Check sheet for the modelled part. Datum: model origin and axes. Units: mm. Coordinates: 2 decimals unless noted, no trailing zeros. Order: outer loops, then holes, each group sorted by start corner. A loop starts at its lowest first (then second) coordinate and runs counter-clockwise, first axis right, second up. Notation, with made-up numbers: (18.25, 62.25) -> (32.25, 62.25) arc R26 ccw to (32.25, 78.25) -> close; hole circle Ø4 at (12, 60.25). An arc over 180 degrees is marked (long way). Put each result on its own line as item: value. Start each with the question number.
Autodesk Inventor part; units mm, degrees
ref_plane "YZ Plane" through (0, 0, 0) normal (1, 0, 0) x (0, 1, 0)
ref_plane "XZ Plane" through (0, 0, 0) normal (0, 1, 0) x (-1, 0, 0)
ref_plane "XY Plane" through (0, 0, 0) normal (0, 0, 1) x (1, 0, 0)
sketch "Náčrt1" plane through (0, 0, 0) normal (0, 0, 1) x (1, 0, 0)
  line L0 (-50, 25) -> (30, 25)
  line L1 (36.6643, -25) -> (-87.5, -25)
  line L2 (30, 25) -> (100, 0)
  line L3 (100, 0) -> (100, -25)
  line L4 (100, -25) -> (36.6643, -25)
  line L5 (-125, 0) -> (137.5, 0)
  line L6 (0, 35) -> (0, -35)
  line L7 (-50, 25) -> (-80, 0)
  line L8 (-80, 0) -> (-80, -25)
  line L9 (-80, -25) -> (-87.5, -25)
  point P0 (0, 0)
  point P1 (-35, 10)
  point P2 (15, 10)
  dimension "d0" = 50
  dimension "d2" = 80
  dimension "d3" = 25
  dimension "d4" = 50
  dimension "d6" = 15
  dimension "d16" = 70
  dimension "d17" = 30
  dimension "d18" = 25
  dimension "d19" = 50
  dimension "d20" = 35
  dimension "d21" = 25
  dimension "d22" = 25
extrude "Vysunutí1" add sketch "Náčrt1" along normal mid plane 4
hole "Díra1" at (-35, 10, 0) at (15, 10, 0) direction (0, 0, -1) diameter 6 end through all both
sketch "Náčrt2" plane through (0, 0, 2) normal (0, 0, 1) x (1, 0, 0)
  line L0 (-80, 0) -> (-80, -25)
  line L1 (-80, -25) -> (100, -25)
  line L2 (100, -25) -> (100, 0)
  point P0 (0, 0)
  point P1 (-40, -15)
  point P2 (60, -15)
  dimension "d23" = 40
  dimension "d24" = 10
  dimension "d25" = 40
  dimension "d26" = 10
hole "Díra2" at (-40, -15, 2) at (60, -15, 2) direction (0, 0, -1) diameter 3 depth 8
properties part number "Trup" material "Dřevo (Bříza)"
1) Sectioned sample at B-B (y = -15). Record the boundary of the cut face in (x, z), plus the area to 3 significant figures.
2) Mould release check, pull along X, two halves, no side actions. Record for faces 1 (the flat face through (-64.79, 12.675, -0.028)), 2 (the flat face through (9, 0, 2)), 3 (the cylindrical face through (17.93, 10.65, -0.03)): +X half, -X half, draft (parallel to the pull), parting line (faces both ways), or undercut.
3) Sectioned sample at C-C (z = -0.2). Record the boundary of the cut face in (x, y).
4) Sectioned sample at A-A (x = 15). Record the boundary of the cut face in (y, z), plus the area to 3 significant figures.
5) Scan lines: line 1 along X through (y, z) = (-15, -0.55); line 2 along Y through (x, z) = (15, -0.05); line 3 along Y through (x, z) = (-40, -0.3). Record each from-to range of solid material in increasing order. Write a range as [from, to].
6) Gauge pin test, flat end, axial feed: pin 1 (1 mm diameter, centred on y = 14.5, z = -1, fed in from -X). Record the tip position at first contact, or that the pin passes through.
7) Sectioned sample at D-D (y = 10). Record the boundary of the cut face in (x, z), plus the area to 3 significant figures.
Entries:
1. outline: (-80, -2) -> (-41.5, -2) -> (-41.5, 2) -> (-80, 2) -> close; (-38.5, -2) -> (58.5, -2) -> (58.5, 2) -> (-38.5, 2) -> close; (61.5, -2) -> (100, -2) -> (100, 2) -> (61.5, 2) -> close
1. area: 696 mm2
2. face 1: -X half
2. face 2: draft
2. face 3: undercut
3. outline: (-80, -25) -> (100, -25) -> (100, 0) -> (30, 25) -> (-50, 25) -> (-80, 0) -> close; hole circle Ø3 at (-40, -15); hole circle Ø6 at (-35, 10); hole circle Ø6 at (15, 10); hole circle Ø3 at (60, -15)
4. outline: (-25, -2) -> (7, -2) -> (7, 2) -> (-25, 2) -> close; (13, -2) -> (25, -2) -> (25, 2) -> (13, 2) -> close
4. area: 176 mm2
5. line 1: x = [-80, -41.5], [-38.5, 58.5], [61.5, 100]
5. line 2: y = [-25, 7], [13, 25]
5. line 3: y = [-25, -16.5], [-13.5, 25]
6. pin 1: stops at x = -63.2
7. outline: (-68, -2) -> (-38, -2) -> (-38, 2) -> (-68, 2) -> close; (-32, -2) -> (12, -2) -> (12, 2) -> (-32, 2) -> close; (18, -2) -> (72, -2) -> (72, 2) -> (18, 2) -> close
7. area: 512 mm2
